```python
from build123d import *

# Parameters (mm, degrees)
F1_R     = 42.509287
F1_R_2   = 33.709002
F2_DEPTH = 6.35
F0_R     = 3.175
F3_DEPTH = 25.4


with BuildPart() as f2:
    # F1 (on Top) → F2 (new body)
    with BuildSketch(Plane.XY):
        Circle(F1_R)
        Circle(F1_R_2, mode=Mode.SUBTRACT)
    extrude(amount=F2_DEPTH)

    # F0 (on Top) → F3 (join)
    with BuildSketch(Plane.XY):
        with Locations((38.1, 0)):
            Circle(F0_R)
        with Locations((36.992883, -9.117927)):
            Circle(F0_R)
        with Locations((33.735875, -17.705953)):
            Circle(F0_R)
        with Locations((28.51826, -25.264973)):
            Circle(F0_R)
        with Locations((21.643267, -31.355685)):
            Circle(F0_R)
        with Locations((13.510446, -35.624119)):
            Circle(F0_R)
        with Locations((4.592448, -37.822208)):
            Circle(F0_R)
        with Locations((-4.592448, -37.822208)):
            Circle(F0_R)
        with Locations((-13.510446, -35.624119)):
            Circle(F0_R)
        with Locations((-21.643267, -31.355685)):
            Circle(F0_R)
        with Locations((-28.51826, -25.264973)):
            Circle(F0_R)
        with Locations((-33.735875, -17.705953)):
            Circle(F0_R)
        with Locations((-36.992883, -9.117927)):
            Circle(F0_R)
        with Locations((-38.1, 0)):
            Circle(F0_R)
        with Locations((-36.992883, 9.117927)):
            Circle(F0_R)
        with Locations((-33.735875, 17.705953)):
            Circle(F0_R)
        with Locations((-28.51826, 25.264973)):
            Circle(F0_R)
        with Locations((-21.643267, 31.355685)):
            Circle(F0_R)
        with Locations((-13.510446, 35.624119)):
            Circle(F0_R)
        with Locations((-4.592448, 37.822208)):
            Circle(F0_R)
        with Locations((4.592448, 37.822208)):
            Circle(F0_R)
        with Locations((13.510446, 35.624119)):
            Circle(F0_R)
        with Locations((21.643267, 31.355685)):
            Circle(F0_R)
        with Locations((28.51826, 25.264973)):
            Circle(F0_R)
        with Locations((33.735875, 17.705953)):
            Circle(F0_R)
        with Locations((36.992883, 9.117927)):
            Circle(F0_R)
    extrude(amount=F3_DEPTH)


solid = f2.part
```
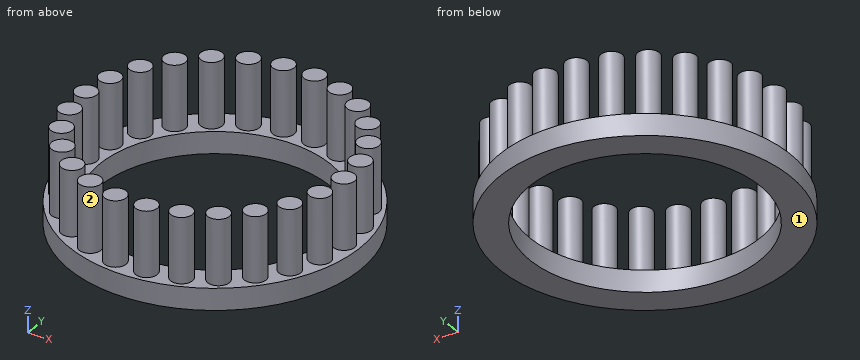
Part model, mm, in its own coordinate system. Face numbers are marked on the shaded views. Round coordinates to 2 decimals unless told otherwise and drop trailing zeros. Order: outer loops, then holes, each group sorted by start corner. A loop starts at its lowest first (then second) coordinate and runs counter-clockwise, first axis right, second up. Notation, with made-up numbers: M 23,25.5 L 53,25.5 A12 cw 53,37.5 Z; hole C 20.25,-22 d11. An arc over 180 degrees is marked long. Answer in a Markdown table with one row per item. Add a question column.
Q1. Cut at D-D on x = 38.1. Give the cut face in (y, z) (3 decimals), and give its area (3 significant figures).
Q2. Cut at C-C on z = 8. Give the number of separate pieces and of enclosed holes in the cut face, and give its area (3 significant figures).
Q3. Cut at A-A on y = 0. Give the cut face in (x, z) (3 decimals).
Q4. Wall check: L1, parallel to Y at x = 31, z = 17; L2, parallel to Y at x = 0, z = 4; L3, parallel to Y at x = -39, z = 6.5. Give the ranges that are in metal, low to high. Write a range as from..to.
Q5. Pin check, flat tips, straight feed: pin 1 (4 mm diameter, centred on x = 9, z = 11.5, fed in from +Y); pin 2 (1 mm diameter, centred on y = -31, z = 6, fed in from +X); pin 3 (1 mm diameter, centred on y = 20.5, z = 3.5, fed in from +X); pin 4 (10 mm diameter, centred on x = 6, y = -26, fed in from -Z). Stop position of each tip, or through.
Q6. Cut at B-B on x = 0. Give the cut face in (y, z).
Q7. Mould opens along Y. For the marked faces 1 and 2 say: +Y half, -Y half, draft (parallel to the pull), parting line (faces both ways), or undercut.
Established:
| question | item | result |
|---|---|---|
| 1 | outline | M -18.853,0 L 18.853,0 L 18.853,6.35 L 12.094,6.35 L 12.094,25.4 L 6.142,25.4 L 6.142,6.35 L 3.175,6.35 L 3.175,25.4 L -3.175,25.4 L -3.175,6.35 L -6.142,6.35 L -6.142,25.4 L -12.094,25.4 L -12.094,6.35 L -18.853,6.35 Z |
| 1 | area | 587 mm2 |
| 2 | separate pieces | 26 |
| 2 | enclosed holes | 0 |
| 2 | area | 823 mm2 |
| 3 | outline | M -42.509,0 L -33.709,0 L -33.709,6.35 L -34.925,6.35 L -34.925,25.4 L -41.275,25.4 L -41.275,6.35 L -42.509,6.35 Z; M 33.709,0 L 42.509,0 L 42.509,6.35 L 41.275,6.35 L 41.275,25.4 L 34.925,25.4 L 34.925,6.35 L 33.709,6.35 Z |
| 4 | L1 | y = -27.25..-23.28, -19.32..-16.09, 16.09..19.32, 23.28..27.25 |
| 4 | L2 | y = -42.51..-33.71, 33.71..42.51 |
| 4 | L3 | y = -11.58..-6.66, -3.04..3.04, 6.66..11.58 |
| 5 | pin 1 | stops at y = 39.89 |
| 5 | pin 2 | stops at x = 29.61 |
| 5 | pin 3 | stops at x = 37.51 |
| 5 | pin 4 | passes through |
| 6 | outline | M -42.51,0 L -33.71,0 L -33.71,6.35 L -42.51,6.35 Z; M 33.71,0 L 42.51,0 L 42.51,6.35 L 33.71,6.35 Z |
| 7 | face 1 | draft |
| 7 | face 2 | undercut |
